Work out the finished part from the listing and answer in its coordinate system (mm). A direction names the side the tool comes from. Round coordinates to 2 decimals unless told otherwise and drop trailing zeros. Order: outer loops, then holes, each group sorted by start corner. A loop starts at its lowest first (then second) coordinate and runs counter-clockwise, first axis right, second up. Notation, with made-up numbers: (-19.75, 31.25) -> (26.25, 31.25) arc R29 cw to (26.25, 55.25) -> close; hole circle Ø9 at (-37, 7). An arc over 180 degrees is marked (long way). Use a Markdown table: item, result. Add a question column.
Item 1: A cutting plane is placed at C-C, the plane y = -6. Determine the outline of the cut face in (x, z), plus the area to 3 significant figures.
Item 2: Find the intervals of material crossed by L1, parallel to Z at x = 0, y = 1.25; L2, parallel to Y at x = 1.25, z = 2.5; L3, parallel to Y at x = 0.75, z = -0.5, in increasing order. Write a range as [from, to].
Item 3: A cutting plane is placed at A-A, the plane z = 0. Determine the outline of the cut face in (x, y), plus the area to 3 significant figures.
Item 4: A flat-ended cylindrical pin translates along its axis: P1, Ø2.5, axis at y = -21.5, z = 0.5, coming from the +X side. Find the tip coordinate at first contact, or state that the pin passes through.
Item 5: A tool of negligible diameter and unlimited length cuts with its end or side. For faces 1 (the flat face through (-3, 0, 0)), 2 (the flat face through (-1, -23.5, 0)), 3 (the cylindrical face through (-0.54, -17.74, -2.44)), 4 (the flat face through (0.6, -21, 0)), from which of +Z, -Z, +X, -X, +Y, -Y can it reach the whole face along a straight path? Write none if from no direction.
Item 6: A cutting plane is placed at B-B, the plane x = 0. Determine the outline of the cut face in (y, z).
Item 7: A cutting plane is placed at D-D, the plane x = 2. Determine the outline of the cut face in (y, z).
from build123d import *

# Parameters (mm, degrees)
F1_DEPTH = 17
F2_R     = 2.5
F3_DEPTH = 1.5
F4_R     = 2.5
F5_DEPTH = 4
F7_DEPTH = 5


with BuildPart() as f1:
    # F0 (on Front) → F1 (new body)
    with BuildSketch(Plane.XZ):
        with BuildLine():
            Line((2.8721443851, -1.9113572746), (2.8721443851, 1.9113572746))
            ThreePointArc((2.8721443851, 1.9113572746), (-3.45, 0), (2.8721443851, -1.9113572746))
        make_face()
    extrude(amount=F1_DEPTH)

    # F2 (on face) → F3 (join)
    with BuildSketch(Plane.XZ.offset(17)):
        Circle(F2_R)
    extrude(amount=F3_DEPTH)

    # F4 (on face) → F5 (join)
    with BuildSketch(Plane(origin=(0, 0, 0), x_dir=(-1, 0, 0), z_dir=(0, 1, 0))):
        Circle(F4_R)
    extrude(amount=F5_DEPTH)

    # F6 (on face) → F7 (join)
    with BuildSketch(Plane.XZ.offset(18.5)):
        with BuildLine():
            Line((0.6, -2.3237900077), (0.6, 2.3237900077))
            ThreePointArc((0.6, 2.3237900077), (-2.4, 0), (0.6, -2.3237900077))
        make_face()
    extrude(amount=F7_DEPTH)


solid = f1.part
Reported:
| question | item | result |
|---|---|---|
| 1 | outline | (2.87, -1.91) -> (2.87, 1.91) arc R3.45 ccw (long way) to start |
| 1 | area | 35.9 mm² |
| 2 | L1 | [-2.5, 2.5] |
| 2 | L2 | [-17, 0] |
| 2 | L3 | [-18.5, 4] |
| 3 | outline | (-3.45, -17) -> (-2.5, -17) -> (-2.5, -18.5) -> (-2.4, -18.5) -> (-2.4, -23.5) -> (0.6, -23.5) -> (0.6, -18.5) -> (2.5, -18.5) -> (2.5, -17) -> (2.87, -17) -> (2.87, 0) -> (2.5, 0) -> (2.5, 4) -> (-2.5, 4) -> (-2.5, 0) -> (-3.45, 0) -> close |
| 3 | area | 150 mm² |
| 4 | P1 | x = 0.6 |
| 5 | face 1 | +Y |
| 5 | face 2 | +Z, -Z, +X, -X, -Y |
| 5 | face 3 | -Y |
| 5 | face 4 | +Z, -Z, +X, -Y |
| 6 | outline | (-23.5, -2.4) -> (-18.5, -2.4) -> (-18.5, -2.5) -> (-17, -2.5) -> (-17, -3.45) -> (0, -3.45) -> (0, -2.5) -> (4, -2.5) -> (4, 2.5) -> (0, 2.5) -> (0, 3.45) -> (-17, 3.45) -> (-17, 2.5) -> (-18.5, 2.5) -> (-18.5, 2.4) -> (-23.5, 2.4) -> close |
| 7 | outline | (-18.5, -1.5) -> (-17, -1.5) -> (-17, -2.81) -> (0, -2.81) -> (0, -1.5) -> (4, -1.5) -> (4, 1.5) -> (0, 1.5) -> (0, 2.81) -> (-17, 2.81) -> (-17, 1.5) -> (-18.5, 1.5) -> close |
